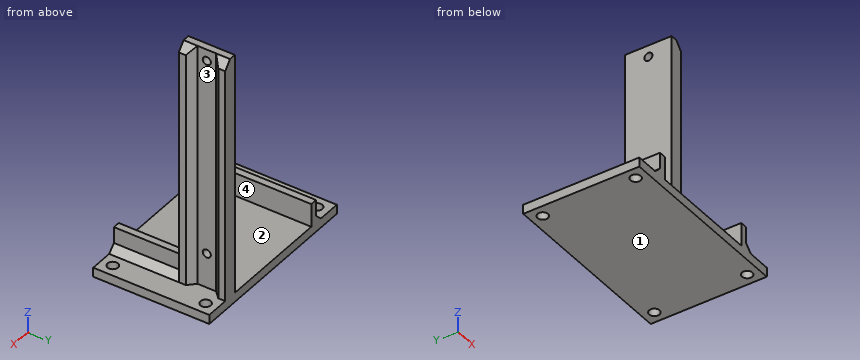
Autodesk Fusion 360 part; units mm, degrees
sketch "Sketch1" plane through (0, 0, 0) normal (0, 1, 0) x (1, 0, 0)
  line L0 (0, 0) -> (-48, 0) construction
  line L1 (-48, 0) -> (-48, -115) construction
  line L2 (-48, -115) -> (0, -115) construction
  line L3 (0, -115) -> (0, 0) construction
  line L4 (0, -105) -> (3, -105)
  line L5 (3, -105) -> (3, 0)
  line L6 (3, 0) -> (16, 0)
  line L7 (16, 0) -> (16, 4)
  line L8 (16, 4) -> (-64, 4)
  line L9 (-64, 4) -> (-64, 0)
  line L10 (-64, 0) -> (-51, 0)
  line L11 (-51, 0) -> (-51, -10)
  line L12 (-51, -10) -> (-48, -10)
  line L13 (-48, -10) -> (-48, 0)
  line L14 (-48, 0) -> (0, 0)
  line L15 (0, 0) -> (0, -105)
  line L16 (0, -100) -> (3, -100) construction
  line L17 (3, -15) -> (0, -14.9007) construction
  line L18 (-51, 0) -> (-48, 0)
  line L19 (0, 0) -> (3, 0)
  line L20 (3, -105) -> (6, -101.4247)
  line L21 (6, -101.4247) -> (6, 0)
  line L22 (0, -10) -> (3, -10)
  dimension "d1" = 48
  dimension "d2" = 115
  dimension "d3" = 3
  dimension "d4" = 4
  dimension "d6" = 13
  dimension "d7" = 13
  dimension "d8" = 10
  dimension "d9" = 15
  dimension "d10" = 85
  dimension "d11" = 5
  dimension "d16" = 3
  dimension "d17" = 140
extrude "Extrude1" add sketch "Sketch1" along normal blind 20 contours L4 L5 L15 L22 | L5 L15 L19 L22 | L6 L7 L8 L9 L10 L14 L18 L19 | L11 L12 L13 L18
extrude "Extrude2" add sketch "Sketch1" against normal blind 30 contours L6 L7 L8 L9 L10 L14 L18 L19
extrude "Extrude3" add sketch "Sketch1" against normal blind 30 contours L5 L15 L19 L22 | L11 L12 L13 L18
sketch "Sketch2" plane through (3, 0, 0) normal (1, 0, 0) x (0, 1, 0)
  line L0 (0, 105) -> (0, 10)
  line L1 (0, 10) -> (-30, 10)
  line L2 (-30, 10) -> (-30, 0)
  line L3 (-30, 0) -> (20, 0)
  line L4 (20, 0) -> (20, 105)
  line L5 (20, 105) -> (0, 105)
  line L6 (10, 105) -> (10, 0) construction
  circle A0 centre (10, 15) radius 1.75
  circle A1 centre (10, 100) radius 1.75
  dimension "d21" = 15
  dimension "d22" = 85
  dimension "d23" = 3.5
extrude "Extrude4" cut sketch "Sketch2" against normal blind 12 contours A0 | A1
extrude "Extrude5" add sketch "Sketch1" along normal blind 3 contours L5 L6 L20 L21
chamfer "Chamfer1" distance 3 angle 45 1 edges at (3, 3, 52.5)
chamfer "Chamfer2" distance 3 angle 45 1 edges at (3, -15, 0)
chamfer "Chamfer3" distance 3 angle 45 1 edges at (-51, -5, 0)
extrude "Extrude6" add sketch "Sketch1" against normal blind 3 from surface at 20 contours L5 L6 L20 L21
chamfer "Chamfer4" distance 3 angle 45 1 edges at (3, 17, 52.5)
sketch "Sketch3" plane through (0, 0, 0) normal (0, 0, 1) x (1, 0, 0)
  line L0 (11, -25) -> (-59, -25) construction
  line L1 (-59, -25) -> (-59, 15) construction
  line L2 (-59, 15) -> (11, 15) construction
  line L3 (11, 15) -> (11, -25) construction
  circle A0 centre (11, -25) radius 2.25
  circle A1 centre (-59, -25) radius 2.25
  circle A2 centre (-59, 15) radius 2.25
  circle A3 centre (11, 15) radius 2.25
  circle A4 centre (11, 15) radius 5 construction
  circle A5 centre (11, -25) radius 5 construction
  circle A6 centre (-59, 15) radius 5 construction
  circle A7 centre (-59, -25) radius 5 construction
  line L4 (-64, -5) -> (20.2305, -5) construction
  line L5 (-64, -30) -> (-64, 20) construction
  line L6 (-24, 20) -> (-24, -32.4373) construction
  line L7 (-48, 20) -> (0, 20) construction
  dimension "d35" = 4.5
  dimension "d36" = 10
  dimension "d37" = 40
  dimension "d38" = 70
extrude "Extrude7" cut sketch "Sketch3" against normal blind 17
equation "d21 = d9"
equation "d22 = d10"
Geometry check sheet. Reference: the model listing, model coordinates, mm. Face numbers are marked on the shaded views. Give positions to 0.01 mm unless a question says otherwise; leave off trailing zeros. Loops run counter-clockwise (first coordinate to the right, second up) from the corner with the lowest first, then second, coordinate; pieces in that order, holes last. Notation, with made-up numbers: M -8,54.5 L 50,54.5 A29 cw 50,81.5 Z; hole C 3,-26 d10. An arc over 180 degrees is marked long. Write each question's results on one line, items separated by ' | '.
1) Release check for a two-part mould opening along X. For the marked faces 1, 2, 3 and 4 record: +X half, -X half, draft (parallel to the pull), parting line (faces both ways), or undercut.
Answers follow:
face 1: draft | face 2: undercut | face 3: +X half | face 4: undercut
2) Section check A-A, the plane y = 10. Record the boundary of the cut face in (x, z), plus the area to 4 significant figures.
Answers follow:
outline: M -64,-4 L 16,-4 L 16,0 L 3,0 L 3,13.25 L 0,13.25 L 0,0 L -48,0 L -48,10 L -51,10 L -51,3 L -54,0 L -64,0 Z; M 0,16.75 L 3,16.75 L 3,98.25 L 0,98.25 Z; M 0,101.75 L 3,101.75 L 3,105 L 0,105 Z | area: 648.5 mm2
3) Section check D-D, the plane y = -8. Record the boundary of the cut face in (x, z).
Answers follow:
outline: M -64,-4 L 16,-4 L 16,0 L 6,0 L 3,3 L 3,10 L 0,10 L 0,0 L -48,0 L -48,10 L -51,10 L -51,3 L -54,0 L -64,0 Z
4) Section check B-B, the plane x = 11. Record the boundary of the cut face in (y, z), plus the area to 3 significant figures.
Answers follow:
outline: M -30,-4 L -27.25,-4 L -27.25,0 L -30,0 Z; M -22.75,-4 L 12.75,-4 L 12.75,0 L -22.75,0 Z; M 17.25,-4 L 20,-4 L 20,0 L 17.25,0 Z | area: 164 mm2
5) Gauge pin test, flat ends, axial feed: pin 1 (5 mm diameter, centred on x = -59, y = 15, fed in from -Z); pin 2 (3 mm diameter, centred on y = -8.5, z = 5.5, fed in from +X); pin 3 (11 mm diameter, centred on x = -59, y = 4.5, fed in from +Z); pin 4 (2 mm diameter, centred on x = -38, y = 13, fed in from +Z). Record the tip position at first contact, or that the pin passes through.
Answers follow:
pin 1: z = -4 | pin 2: x = 3 | pin 3: z = 0.5 | pin 4: z = 0
6) Thickness scan on line 1 (Y direction, x = -59, z = -2.05); line 2 (Z direction, x = 1.85, y = 10); line 3 (X direction, y = 7, z = 81). Record the ranges inside material, lowest first.
Answers follow:
line 1: -30 to -27.25, -22.75 to 12.75, 17.25 to 20 | line 2: -4 to 13.25, 16.75 to 98.25, 101.75 to 105 | line 3: 0 to 3
